Read the model definition and answer for the solid it produces. Units are mm, in the model's axes. Coordinates: 2 decimals unless noted, no trailing zeros. Write each loop counter-clockwise with the first axis right and the second up, starting at its lowest first coordinate (ties: lowest second). Pieces come first, ordered by that corner, then holes.
(1) Section B-B on z = 0 is taken. Write down the section's boundary in (x, y).
(2) Section A-A on x = 0 is taken. Write down the section's boundary in (y, z).
(3) Find the intervals of material crossed by probe 1 along X at (y, z) = (1.75, 0); probe 2 along Z at (x, y) = (-0.75, 1.5), in increasing order.
(4) The mould has two halves that part along X. Classify faces 1 (the cylindrical face through (-1.19, 1.26, 5.37)), 2 (the flat face through (-3, 0, 3)), 3 (the cylindrical face through (-3.746, 1.263, -0.165)): +X half, -X half, draft (parallel to the pull), parting line (faces both ways), or undercut.
(5) Given pin 1 (1.5 mm diameter, centred on x = 4, y = 1, fed in from +Z), flat-ended and moving along its own axis, determine where the tip first touches the part or whether it passes through.
(6) Section C-C on y = 0.9 is taken. Write down the section's boundary in (x, z), then the cut area to 3 significant figures.
from build123d import *

# Parameters (mm, degrees)
SKETCH_1_W = 1.75
SKETCH_1_H = 2.5
FILLET_1_R = 0.3


with BuildPart() as part:
    # Эскиз1 → Повернуть1 (revolve)
    with BuildSketch(Plane.XY):
        with Locations((4.625, 1.25)):
            Rectangle(SKETCH_1_W, SKETCH_1_H)
    revolve(axis=Axis((0, 0, 0), (0, 1, 0)))

    # Скругление1
    fillet_1_edges = [part.edges().sort_by_distance(p)[0] for p in [
        (-5.5, 0, 0),
        (-5.5, 2.5, 0),
        (-3.75, 2.5, 0),
        (-3.75, 0, 0),
    ]]
    fillet(fillet_1_edges, radius=FILLET_1_R)


solid = part.part
Response:
1. outline: (-5.5, 0.3) arc R0.3 ccw to (-5.2, 0) - (-4.05, 0) arc R0.3 ccw to (-3.75, 0.3) - (-3.75, 2.2) arc R0.3 ccw to (-4.05, 2.5) - (-5.2, 2.5) arc R0.3 ccw to (-5.5, 2.2) - close; (3.75, 0.3) arc R0.3 ccw to (4.05, 0) - (5.2, 0) arc R0.3 ccw to (5.5, 0.3) - (5.5, 2.2) arc R0.3 ccw to (5.2, 2.5) - (4.05, 2.5) arc R0.3 ccw to (3.75, 2.2) - close
2. outline: (0, -5.2) arc R0.3 ccw to (0.3, -5.5) - (2.2, -5.5) arc R0.3 ccw to (2.5, -5.2) - (2.5, -4.05) arc R0.3 ccw to (2.2, -3.75) - (0.3, -3.75) arc R0.3 ccw to (0, -4.05) - close; (0, 4.05) arc R0.3 ccw to (0.3, 3.75) - (2.2, 3.75) arc R0.3 ccw to (2.5, 4.05) - (2.5, 5.2) arc R0.3 ccw to (2.2, 5.5) - (0.3, 5.5) arc R0.3 ccw to (0, 5.2) - close
3. probe 1: x = -5.5 to -3.75, 3.75 to 5.5
3. probe 2: z = -5.45 to -3.67, 3.67 to 5.45
4. face 1: parting line
4. face 2: draft
4. face 3: undercut
5. pin 1: stops at z = 4.44
6. outline: circle Ø11 at (0, 0); hole circle Ø7.5 at (0, 0)
6. area: 50.9 mm2
